Verification items for the finished model (mm, model axes). A direction names the side the tool comes from. Round coordinates to 2 decimals unless told otherwise and drop trailing zeros. Write each loop counter-clockwise with the first axis right and the second up, starting at its lowest first coordinate (ties: lowest second). Pieces come first, ordered by that corner, then holes. Notation, with made-up numbers: M -15,-31 L 33,-31 A29 ccw 33,-1 Z; hole C -15,46 d4. An arc over 180 degrees is marked long. One line per item, written item: value. Start each with the question number.
from build123d import *

# Parameters (mm, degrees)
SKETCH_2_R          = 1.4
CUT_EXTRUDE_1_DEPTH = 50.451996926


with BuildPart() as part:
    # 草图1 → 旋转1 (revolve)
    with BuildSketch(Plane.XY):
        Polygon((0, 0), (-3.5, 0), (-3.5, 6), (-7.75, 6), (-7.75, 42.8), (-14.5, 42.8), (-14.5, 45), (0, 45), align=None)
    revolve(axis=Axis((0, 45, 0), (0, -1, 0)))

    # 草图2 → 切除-拉伸1 (cut, through all)
    with BuildSketch(Plane(origin=(0, 45, 0), x_dir=(1, 0, 0), z_dir=(0, 1, 0))):
        with Locations(Location((0, 12, 0), (0, 0, 180))):
            Circle(SKETCH_2_R)
        with Locations(Location((10.392304845, -6, 0), (0, 0, 180))):
            Circle(SKETCH_2_R)
        with Locations(Location((-10.392304845, -6, 0), (0, 0, 180))):
            Circle(SKETCH_2_R)
    extrude(amount=-CUT_EXTRUDE_1_DEPTH, mode=Mode.SUBTRACT)


solid = part.part
1) Cross-section at A-A (x = -0.25). Record the boundary of the cut face in (y, z), then the cut area to 3 significant figures.
2) Cross-section at D-D (x = 10.25). Record the boundary of the cut face in (y, z).
3) Thickness scan on line 1 (Y direction, x = 1.5, z = -9.25); line 2 (Z direction, x = 0, y = 40.5); line 3 (Y direction, x = 5.25, z = -2.25). Record the ranges inside material, lowest first.
4) Cross-section at B-B (z = 6). Record the boundary of the cut face in (x, y).
5) Cross-section at C-C (z = -12). Record the boundary of the cut face in (x, y), then the cut area to 3 significant figures.
6) Gauge pin test, flat ends, axial feed: pin 1 Ø4 at (x, z) = (2, 7.5) entering from -Y; pin 2 Ø2 at (x, y) = (6, 36) entering from -Z; pin 3 Ø8 at (y, z) = (40.5, -7.5) entering from -X. Record the tip position at first contact, or that the pin passes through.
7) Mould release check, pull along X, two halves, no side actions. Record for faces 3 (the cylindrical face through (-9.36, 43.915, 6.946)), 4 (the cylindrical face through (-6.691, 43.915, 12.864)), 5 (the cylindrical face through (-0.75, 43.92, -10.82)), 6 (the flat face through (0, 0, 0)): pulls with the +X half, pulls with the -X half, needs draft (parallel to the pull), parting line crosses it, or undercut.
8) Access from +Z, -Z, +X, -X, +Y, -Y to the whole of each face (thin tool, end or side, straight path). Record for faces 1 (the flat face through (0, 45, 0)), 2 (the flat face through (6, 42.8, 6)).
Results below:
1. outline: M 0,-3.49 L 6,-3.49 L 6,-7.75 L 42.8,-7.75 L 42.8,-10.62 L 45,-10.62 L 45,14.5 L 42.8,14.5 L 42.8,7.75 L 6,7.75 L 6,3.49 L 0,3.49 Z; M 42.8,-14.5 L 45,-14.5 L 45,-13.38 L 42.8,-13.38 Z
1. area: 670 mm²
2. outline: M 42.8,-10.26 L 45,-10.26 L 45,4.61 L 42.8,4.61 Z; M 42.8,7.39 L 45,7.39 L 45,10.26 L 42.8,10.26 Z
3. line 1: y = 42.8 to 45
3. line 2: z = -7.75 to 7.75
3. line 3: y = 6 to 45
4. outline: M -13.2,42.8 L -11.79,42.8 L -11.79,45 L -13.2,45 Z; M -8.99,42.8 L -4.91,42.8 L -4.91,6 L 4.91,6 L 4.91,42.8 L 8.99,42.8 L 8.99,45 L -8.99,45 Z; M 11.79,42.8 L 13.2,42.8 L 13.2,45 L 11.79,45 Z
5. outline: M -8.14,42.8 L -1.4,42.8 L -1.4,45 L -8.14,45 Z; M 1.4,42.8 L 8.14,42.8 L 8.14,45 L 1.4,45 Z
5. area: 29.7 mm²
6. pin 1: stops at y = 6
6. pin 2: stops at z = -5.92
6. pin 3: stops at x = -13.87
7. face 3: undercut
7. face 4: parting line crosses it
7. face 5: undercut
7. face 6: needs draft
8. face 1: +Z, -Z, +X, -X, +Y
8. face 2: -Y
